Here's the drawing with two shaded views (mm, measured from the low corner). I have some questions. A direction names the side the tool comes from. Coordinates: 2 decimals unless noted, no trailing zeros. Write each loop counter-clockwise with the first axis right and the second up, starting at its lowest first coordinate (ties: lowest second). Pieces come first, ordered by that corner, then holes. Notation, with made-up numbers: (-5.75, 4.5) -> (21.25, 4.5) arc R26 cw to (21.25, 35.5) -> close; hole circle Ø7 at (21.5, 66.25). An arc over 180 degrees is marked (long way). Put each result on its own line as item: value. Start each with the question number.
Item 1: On a 3-axis mill with a long thin cutter (end or side, diameter ignored), from which of +Z, -Z, +X, -X, +Y, -Y can I reach the whole of each face in a straight line? I mean the marked faces 1 and 2. Say none if no direction works.
Item 2: I want a section at B-B, the plane z = 119. List the corners of the cut face in (x, y) for me.
Item 3: I want a section at C-C, the plane y = 19. List the corners of the cut face in (x, z) for me.
Item 4: I want a section at A-A, the plane x = 161. List the corners of the cut face in (y, z) for me.
Item 5: I need wall thicknesses on line 1 (Z direction, x = 86.5, y = 8); line 2 (X direction, y = 6, z = 153); line 3 (Z direction, x = 167.5, y = 5.5). Which ranges of each line are inside material? Lowest first, please. Write a range as [from, to].
Item 6: For pin 1 (5.5 mm diameter, centred on x = 62, y = 7, fed in from -Z); pin 2 (1.5 mm diameter, centred on y = 7, z = 138.5, fed in from -X); pin 3 (5 mm diameter, centred on x = 62, y = 5, fed in from +Z), each with a flat end and sliding along its axis, tell me the tip position at first contact or that it passes through.
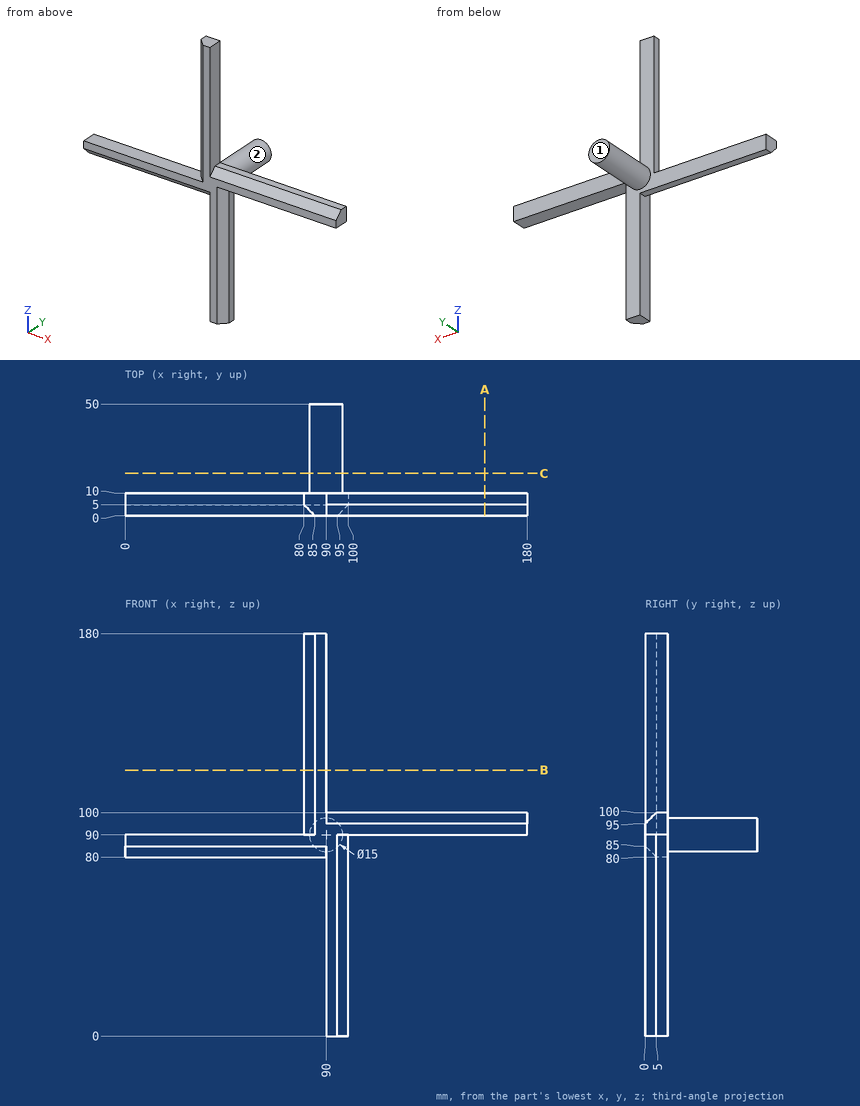
Calculated:
1. face 1: +Z, -Z, +X, -X, +Y
1. face 2: +Y
2. outline: (80, 5) -> (85, 0) -> (90, 0) -> (90, 10) -> (80, 10) -> close
3. outline: circle Ø15 at (90, 90)
4. outline: (0, 90) -> (10, 90) -> (10, 100) -> (5, 100) -> (0, 95) -> close
5. line 1: z = [80, 180]
5. line 2: x = [80, 90]
5. line 3: z = [90, 100]
6. pin 1: stops at z = 80
6. pin 2: stops at x = 80
6. pin 3: stops at z = 90
